The model under review builds one solid part; all positions refer to its coordinate system, in mm. A direction names the side the tool comes from. Coordinates: 2 decimals unless noted, no trailing zeros. Order: outer loops, then holes, each group sorted by start corner. A loop starts at its lowest first (then second) coordinate and runs counter-clockwise, first axis right, second up. Notation, with made-up numbers: (48.5, -9) -> (59.5, -9) arc R18 ccw to (59.5, -1) -> close; hole circle Ø5 at (44.5, 65.25). An arc over 180 degrees is marked (long way). Use CSV: the item, a comma, the result in double quotes. Start each with the question number.
```python
from build123d import *

# Parameters (mm, degrees)
F0_W     = 40
F0_H     = 40
F1_DEPTH = 60
F2_T     = -2
F4_D     = 3
F4_DEPTH = 2
F4_TIP   = 0.9012909285
F5_R     = 0.1
F6_R     = 0.1
F8_D     = 3
F8_DEPTH = 2
F8_TIP   = 0.9012909285


with BuildPart() as f1:
    # F0 (on Right) → F1 (new body)
    with BuildSketch(Plane.YZ):
        Rectangle(F0_W, F0_H)
    extrude(amount=F1_DEPTH)

    # F2
    f2_openings = [f1.faces().sort_by_distance(p)[0] for p in [
        (60, 0, 0),
        (0, 0, 0),
    ]]
    offset(amount=F2_T, openings=f2_openings)

    # F4
    with Locations(Plane.XZ.offset(20)):
        with Locations((17.5, 12.5), (42.5, 12.5), (42.5, -12.5), (17.5, -12.5)):
            Hole(F4_D / 2, depth=F4_DEPTH)
            with Locations((0, 0, -(F4_DEPTH + F4_TIP / 2))):  # 118° drill point
                Cone(0, F4_D / 2, F4_TIP, mode=Mode.SUBTRACT)

    # F5
    f5_edges = [f1.edges().sort_by_distance(p)[0] for p in [
        (30, -20, 20),
        (30, 20, 20),
        (30, -20, -20),
        (30, 20, -20),
    ]]
    fillet(f5_edges, radius=F5_R)

    # F6
    f6_edges = [f1.edges().sort_by_distance(p)[0] for p in [
        (30, -18, 18),
        (30, 18, 18),
        (30, -18, -18),
        (30, 18, -18),
    ]]
    fillet(f6_edges, radius=F6_R)

    # F8
    with Locations(Plane(origin=(0, 20, 0), x_dir=(-1, 0, 0), z_dir=(0, 1, 0))):
        with Locations((-39, 12), (-21, -12)):
            Hole(F8_D / 2, depth=F8_DEPTH)
            with Locations((0, 0, -(F8_DEPTH + F8_TIP / 2))):  # 118° drill point
                Cone(0, F8_D / 2, F8_TIP, mode=Mode.SUBTRACT)


solid = f1.part
```
Q1. Add section C-C, the plane x = 17.5. State the section outline as (y, z) points, then the cut area to 3 significant figures.
Q2. Add section A-A, the plane z = 1.5. State the section outline as (x, y) points, then the cut area to 3 significant figures.
Q3. Clearance check with flat-ended pins moving along their axes: pin 1 Ø4 at (x, z) = (17.5, -12.5) entering from -Y; pin 2 Ø1.8 at (x, z) = (39, 12) entering from +Y. State where each tip first meets the part, or that it passes through.
Q4. Add section D-D, the plane x = 55. State the section outline as (y, z) points, then the cut area to 3 significant figures.
Q5. To check wall thickness, follow probe 1 along Z at (x, y) = (42.5, -18.5); probe 2 along Z at (x, y) = (5.5, 2); probe 3 along X at (y, z) = (19.55, -12). State the ranges of each line that lie inside material, in increasing order.
Q6. For faces 1 (the cylindrical face through (44, -18.99, -12.43)), 2 (the flat face through (30, 0, -20)), 3 (the flat face through (30, 18, 0)), 4 (the flat face through (0, -2, -19)), 5 (the cylindrical face through (37.8, 19, 11.1)), list the 3-axis set-ups (+Z, -Z, +X, -X, +Y, -Y) from which the entire face can be reached by the end or side of a thin tool; tool diameter is ignored.
Q7. Draft analysis for pull direction X (two halves, no side actions). For faces 6 (the flat face through (60, -2, -19)), 7 (the flat face through (30, -18, 0)), 8 (the cylindrical face through (19, -18.99, 12.57)), state which applies: +X half, -X half, draft (parallel to the pull), parting line (faces both ways), or undercut.
Answer block:
1,outline,"(-20, -19.9) arc R0.1 ccw to (-19.9, -20) -> (19.9, -20) arc R0.1 ccw to (20, -19.9) -> (20, 19.9) arc R0.1 ccw to (19.9, 20) -> (-19.9, 20) arc R0.1 ccw to (-20, 19.9) -> (-20, 14) -> (-18, 14) -> (-18, 17.9) arc R0.1 cw to (-17.9, 18) -> (17.9, 18) arc R0.1 cw to (18, 17.9) -> (18, -17.9) arc R0.1 cw to (17.9, -18) -> (-17.9, -18) arc R0.1 cw to (-18, -17.9) -> (-18, -14) -> (-20, -14) -> close; (-20, -11) -> (-18, -11) -> (-18, 11) -> (-20, 11) -> close"
1,area,"292 mm²"
2,outline,"(0, -20) -> (60, -20) -> (60, -18) -> (0, -18) -> close; (0, 18) -> (60, 18) -> (60, 20) -> (0, 20) -> close"
2,area,"240 mm²"
3,pin 1,"stops at y = -20"
3,pin 2,"stops at y = -18"
4,outline,"(-20, -19.9) arc R0.1 ccw to (-19.9, -20) -> (19.9, -20) arc R0.1 ccw to (20, -19.9) -> (20, 19.9) arc R0.1 ccw to (19.9, 20) -> (-19.9, 20) arc R0.1 ccw to (-20, 19.9) -> close; hole (-18, -17.9) arc R0.1 ccw to (-17.9, -18) -> (17.9, -18) arc R0.1 ccw to (18, -17.9) -> (18, 17.9) arc R0.1 ccw to (17.9, 18) -> (-17.9, 18) arc R0.1 ccw to (-18, 17.9) -> close"
4,area,"304 mm²"
5,probe 1,"z = -20 to -14, -11 to 11, 14 to 20"
5,probe 2,"z = -20 to -18, 18 to 20"
5,probe 3,"x = 0 to 19.5, 22.5 to 60"
6,face 1,"-Y"
6,face 2,"-Z, +X, -X, +Y, -Y"
6,face 3,"+X, -X"
6,face 4,"+Z, -Z, -X, +Y, -Y"
6,face 5,"+Y"
7,face 6,"+X half"
7,face 7,"draft"
7,face 8,"undercut"
